Source: CAD feature listing. Evaluate the final solid. Frame: model axes, mm. A direction names the side the tool comes from. Round coordinates to 2 decimals unless told otherwise and drop trailing zeros. Order: outer loops, then holes, each group sorted by start corner. A loop starts at its lowest first (then second) coordinate and runs counter-clockwise, first axis right, second up. Notation, with made-up numbers: (18.5, -33.75) -> (44.5, -33.75) arc R7 cw to (44.5, -29.75) -> close; hole circle Ø2 at (3, 31). An arc over 180 degrees is marked (long way). One line per item, written item: value. Start each with the question number.
1) Section D-D (x = 31). Return the cut outline in (y, z).
2) Section A-A (y = -115). Return the cut outline in (x, z), and give its area (3 significant figures).
3) Mould query, pull axis Y, two halves, no side actions, for faces 6 (the face through (48.979, -64, 7)), 7 (the face through (5.681, -11.206, 1.479)), 8 (the face through (5.681, -111.206, 1.479)), 9 (the face through (24, -130, 6)). Classes: pulls with the +Y half, pulls with the -Y half, needs draft (parallel to the pull), parting line crosses it, or undercut.
4) Reachability of faces 1 (the face through (7, -64, 3)), 2 (the face through (21.858, -64.09, 2.795)), 3 (the face through (9, -64, 0)), 4 (the face through (34, -64, 9)), 5 (the face through (37, -64, 6)) from +Z, -Z, +X, -X, +Y, -Y: full face, straight path, thin tool, end or side. Return the list, or none.
5) Section C-C (y = -45). Return the cut outline in (x, z).
6) Section B-B (x = 8.1). Return the cut outline in (y, z), and give its area (3 significant figures).
7) Pin query (flat end, axial travel): P1, Ø5, axis at x = 35, y = -19.5, coming from the -Z side; P2, Ø14.5, axis at x = 8.1, y = -115, coming from the +Z side; P3, Ø4, axis at y = -25, z = 8, coming from the -X side. Return the tip coordinate at first contact, or that it passes through.
8) Ray query, L1, parallel to Y at x = 8.1, z = 0.8; L2, parallel to X at y = -124, z = 1; L3, parallel to Y at x = 4, z = 2. Return the intervals inside material, ascending.
```python
from build123d import *

# Parameters (mm, degrees)
F1_DEPTH = 130
F3_D     = 9
F4_D     = 9


with BuildPart() as f1:
    # F0 (on Front) → F1 (new body)
    with BuildSketch(Plane.XZ):
        with BuildLine():
            Line((48.978579, 9), (18.978579, 9))
            ThreePointArc((18.978579, 9), (16.111115, 7.855998), (14.818609, 5.052336))
            Line((14.818609, 5.052336), (14.735883, 3.473832))
            ThreePointArc((14.735883, 3.473832), (14.580745, 3.137313), (14.236568, 3))
            Line((14.236568, 3), (0.5, 3))
            ThreePointArc((0.5, 3), (0.146447, 2.853553), (0, 2.5))
            Line((0, 2.5), (0, 0.5))
            ThreePointArc((0, 0.5), (0.146447, 0.146447), (0.5, 0))
            Line((0.5, 0), (17.240685, 0))
            ThreePointArc((17.240685, 0), (17.584863, 0.137313), (17.74, 0.473832))
            Line((17.74, 0.473832), (17.979949, 5.052336))
            ThreePointArc((17.979949, 5.052336), (18.290224, 5.725374), (18.978579, 6))
            Line((18.978579, 6), (20.74132, 6))
            ThreePointArc((20.74132, 6), (21.429674, 5.725374), (21.739949, 5.052336))
            Line((21.739949, 5.052336), (21.979898, 0.473832))
            ThreePointArc((21.979898, 0.473832), (22.135036, 0.137313), (22.479213, 0))
            Line((22.479213, 0), (24.500685, 0))
            ThreePointArc((24.500685, 0), (24.844863, 0.137313), (25, 0.473832))
            Line((25, 0.473832), (25.239949, 5.052336))
            ThreePointArc((25.239949, 5.052336), (25.550224, 5.725374), (26.238579, 6))
            Line((26.238579, 6), (48.978579, 6))
            Line((48.978579, 6), (48.978579, 9))
        make_face()
    extrude(amount=F1_DEPTH)

    # F3 (through all)
    with Locations(Plane.XY.offset(3)):
        with Locations((8.1, -15)):
            Hole(F3_D / 2)

    # F4 (through all)
    with Locations(Plane.XY.offset(3)):
        with Locations((8.1, -115)):
            Hole(F4_D / 2)


solid = f1.part
```
Findings:
1. outline: (-130, 6) -> (0, 6) -> (0, 9) -> (-130, 9) -> close
2. outline: (0, 0.5) arc R0.5 ccw to (0.5, 0) -> (3.6, 0) -> (3.6, 3) -> (0.5, 3) arc R0.5 ccw to (0, 2.5) -> close; (12.6, 0) -> (17.24, 0) arc R0.5 ccw to (17.74, 0.47) -> (17.98, 5.05) arc R1 cw to (18.98, 6) -> (20.74, 6) arc R1 cw to (21.74, 5.05) -> (21.98, 0.47) arc R0.5 ccw to (22.48, 0) -> (24.5, 0) arc R0.5 ccw to (25, 0.47) -> (25.24, 5.05) arc R1 cw to (26.24, 6) -> (48.98, 6) -> (48.98, 9) -> (18.98, 9) arc R4.17 ccw to (14.82, 5.05) -> (14.74, 3.47) arc R0.5 cw to (14.24, 3) -> (12.6, 3) -> close
2. area: 155 mm2
3. face 6: needs draft
3. face 7: undercut
3. face 8: undercut
3. face 9: pulls with the -Y half
4. face 1: +Z, -X, +Y, -Y
4. face 2: -Z, +Y, -Y
4. face 3: -Z, +X, -X, +Y, -Y
4. face 4: +Z, +X, -X, +Y, -Y
4. face 5: -Z, +X, +Y, -Y
5. outline: (0, 0.5) arc R0.5 ccw to (0.5, 0) -> (17.24, 0) arc R0.5 ccw to (17.74, 0.47) -> (17.98, 5.05) arc R1 cw to (18.98, 6) -> (20.74, 6) arc R1 cw to (21.74, 5.05) -> (21.98, 0.47) arc R0.5 ccw to (22.48, 0) -> (24.5, 0) arc R0.5 ccw to (25, 0.47) -> (25.24, 5.05) arc R1 cw to (26.24, 6) -> (48.98, 6) -> (48.98, 9) -> (18.98, 9) arc R4.17 ccw to (14.82, 5.05) -> (14.74, 3.47) arc R0.5 cw to (14.24, 3) -> (0.5, 3) arc R0.5 ccw to (0, 2.5) -> close
6. outline: (-130, 0) -> (-119.5, 0) -> (-119.5, 3) -> (-130, 3) -> close; (-110.5, 0) -> (-19.5, 0) -> (-19.5, 3) -> (-110.5, 3) -> close; (-10.5, 0) -> (0, 0) -> (0, 3) -> (-10.5, 3) -> close
6. area: 336 mm2
7. P1: z = 6
7. P2: z = 6.88
7. P3: x = 14.98
8. L1: -130 to -119.5, -110.5 to -19.5, -10.5 to 0
8. L2: 0 to 17.77, 21.95 to 25.03
8. L3: -130 to -116.85, -113.15 to -16.85, -13.15 to 0
